Build history of the part. All positions in model axes, mm. A direction names the side the tool comes from. Give positions to 0.01 mm unless a question says otherwise; leave off trailing zeros. Write each loop counter-clockwise with the first axis right and the second up, starting at its lowest first coordinate (ties: lowest second). Pieces come first, ordered by that corner, then holes. Notation, with made-up numbers: M 68.25,26 L 91.25,26 A32 cw 91.25,52 Z; hole C 13,35 d6. An arc over 180 degrees is marked long. Return JSON: item names as keys, results as strings. Group by question number.
Q1. Band-saw the part on C-C, the plane y = 15. Give the cut face in (x, z), then the cut area to 3 significant figures.
Q2. Flat gauge pins, fed straight in: pin 1 Ø2 at (y, z) = (4, -0.5) entering from -X; pin 2 Ø3 at (x, z) = (-14, -0.5) entering from +Y; pin 3 Ø1.5 at (x, z) = (-30.5, 0) entering from +Y. Where does each tip first touch, or does it go through?
Q3. Band-saw the part on D-D, the plane z = 0.7. Give the cut face in (x, y), then the cut area to 3 significant figures.
Q4. Tool access for faces 4 (the flat face through (0, 2, 0)), 5 (the flat face through (-30, 7.5, 0)), 6 (the flat face through (30, 17, 0)): list every direction of +Z, -Z, +X, -X, +Y, -Y with a clear straight run to the whole face (end or side of a thin tool).
Q5. Wall check: probe 1 along Z at (x, y) = (12.5, 2.5); probe 2 along Y at (x, z) = (-5.5, -0.85); probe 3 along X at (y, z) = (5, -0.05). Give the ranges that are in metal, low to high.
Q6. Band-saw the part on A-A, the plane x = 10.5. Give the cut face in (y, z).
Q7. Pull direction Z, two halves, no side cores. Call faces 1 (the flat face through (0, 0, 0)), 2 (the cylindrical face through (26.5, 2.5, 0)), 3 (the cylindrical face through (-28.513, 5.472, -0.195)): +Z half, -Z half, draft (parallel to the pull), parting line (faces both ways), or undercut.
Q8. Band-saw the part on B-B, the plane y = 5.5. Give the cut face in (x, z).
from build123d import *

# Parameters (mm, degrees)
EXTRUDE_1_DEPTH     = 3
EXTRUDE_2_DEPTH     = 0.5
SKETCH_3_R          = 1.5
EXTRUDE_3_DEPTH     = 4.5
EXTRUDE_4_DEPTH     = 10
SKETCH_3_3_R        = 1.5
EXTRUDE_5_DEPTH     = 14
CUT_EXTRUDE_1_DEPTH = 1


with BuildPart() as part:
    # Эскиз1 → Бобышка-Вытянуть1 (new body)
    with BuildSketch(Plane(origin=(0, 0, 0), x_dir=(1, 0, 0), z_dir=(0, 1, 0))):
        with BuildLine():
            Line((30, -2.5), (-30, -2.5))
            ThreePointArc((-30, -2.5), (-32.5, 0), (-30, 2.5))
            Line((-30, 2.5), (30, 2.5))
            ThreePointArc((30, 2.5), (32.5, 0), (30, -2.5))
        make_face()
    extrude(amount=EXTRUDE_1_DEPTH)

    # Эскиз2 → Бобышка-Вытянуть2 (add)
    with BuildSketch(Plane(origin=(0, 3, 0), x_dir=(1, 0, 0), z_dir=(0, 1, 0))):
        with BuildLine():
            ThreePointArc((-30, -2.5), (-28.232233047, -1.767766953), (-27.5, 0))
            ThreePointArc((-27.5, 0), (-28.232233047, 1.767766953), (-30, 2.5))
            ThreePointArc((-30, 2.5), (-32.5, 0), (-30, -2.5))
        make_face()
    extrude(amount=EXTRUDE_2_DEPTH)

    # Эскиз3 → Бобышка-Вытянуть3 (add)
    with BuildSketch(Plane(origin=(0, 3, 0), x_dir=(1, 0, 0), z_dir=(0, 1, 0))):
        with Locations(Location((-30, 0, 0), (0, 0, 270))):
            Circle(SKETCH_3_R)
    extrude(amount=EXTRUDE_3_DEPTH)

    # Эскиз2<3> → Бобышка-Вытянуть4 (add)
    with BuildSketch(Plane(origin=(0, 3, 0), x_dir=(1, 0, 0), z_dir=(0, 1, 0))):
        with BuildLine():
            ThreePointArc((30, -2.5), (31.767766953, -1.767766953), (32.5, 0))
            ThreePointArc((32.5, 0), (31.767766953, 1.767766953), (30, 2.5))
            ThreePointArc((30, 2.5), (27.5, 0), (30, -2.5))
        make_face()
    extrude(amount=EXTRUDE_4_DEPTH)

    # Эскиз3<3> → Бобышка-Вытянуть5 (add)
    with BuildSketch(Plane(origin=(0, 3, 0), x_dir=(1, 0, 0), z_dir=(0, 1, 0))):
        with Locations(Location((30, 0, 0), (0, 0, 270))):
            Circle(SKETCH_3_3_R)
    extrude(amount=EXTRUDE_5_DEPTH)

    # Эскиз4 → Вырез-Вытянуть1 (cut)
    with BuildSketch(Plane(origin=(0, 3, 0), x_dir=(1, 0, 0), z_dir=(0, 1, 0))):
        with BuildLine():
            Line((25, -1.5), (-25, -1.5))
            ThreePointArc((-25, -1.5), (-26.5, 0), (-25, 1.5))
            Line((-25, 1.5), (25, 1.5))
            ThreePointArc((25, 1.5), (26.5, 0), (25, -1.5))
        make_face()
    extrude(amount=-CUT_EXTRUDE_1_DEPTH, mode=Mode.SUBTRACT)


solid = part.part
From the geometry:
{
 "1": {"outline": "C 30,0 d3", "area": "7.07 mm^2"},
 "2": {"pin 1": "stops at x = -32.5", "pin 2": "stops at y = 3", "pin 3": "stops at y = 7.5"},
 "3": {"outline": "M -32.4,0 L 32.4,0 L 32.4,13 L 31.33,13 L 31.33,17 L 28.67,17 L 28.67,13 L 27.6,13 L 27.6,3 L 26.33,3 L 26.33,2 L -26.33,2 L -26.33,3 L -27.6,3 L -27.6,3.5 L -28.67,3.5 L -28.67,7.5 L -31.33,7.5 L -31.33,3.5 L -32.4,3.5 Z", "area": "213 mm^2"},
 "4": {"face 4": "+Y", "face 5": "+Z, -Z, -X, +Y", "face 6": "+Z, -Z, +X, -X, +Y"},
 "5": {"probe 1": "z = -2.5 to -1.5, 1.5 to 2.5", "probe 2": "y = 0 to 2", "probe 3": "x = -31.5 to -28.5, 27.5 to 32.5"},
 "6": {"outline": "M 0,-2.5 L 3,-2.5 L 3,-1.5 L 2,-1.5 L 2,1.5 L 3,1.5 L 3,2.5 L 0,2.5 Z"},
 "7": {"face 1": "draft", "face 2": "undercut", "face 3": "parting line"},
 "8": {"outline": "C -30,0 d3; C 30,0 d5"}
}
